Model file for the job. Use its own axes, mm. Face numbers are marked on the shaded views. A direction names the side the tool comes from. Round coordinates to 2 decimals unless told otherwise and drop trailing zeros. Write each loop counter-clockwise with the first axis right and the second up, starting at its lowest first coordinate (ties: lowest second). Pieces come first, ordered by that corner, then holes.
```python
from build123d import *

# Parameters (mm, degrees)
F0_W     = 50.8
F0_H     = 88.9
F1_DEPTH = 101.6
F2_W     = 50.8
F2_H     = 19.05
F3_DEPTH = 63.5
F4_W     = 50.8
F4_H     = 6.9018518552
F5_DEPTH = 50.8
F6_R     = 5.08


with BuildPart() as f1:
    # F0 (on Top) → F1 (new body)
    with BuildSketch(Plane.XY):
        Rectangle(F0_W, F0_H)
    extrude(amount=F1_DEPTH)

    # F2 (on face) → F3 (cut)
    with BuildSketch(Plane.XY.offset(101.6)):
        with Locations((0, -34.925)):
            Rectangle(F2_W, F2_H)
        with Locations((0, 34.925)):
            Rectangle(F2_W, F2_H)
    extrude(amount=-F3_DEPTH, mode=Mode.SUBTRACT)

    # F4 (on face) → F5 (cut)
    with BuildSketch(Plane.YZ.offset(25.4)):
        with Locations((0, 3.4509259276)):
            Rectangle(F4_W, F4_H)
    extrude(amount=-F5_DEPTH, mode=Mode.SUBTRACT)

    # F6
    f6_edges = [f1.edges().sort_by_distance(p)[0] for p in [
        (0, -25.4, 101.6),
        (-25.4, 0, 101.6),
        (0, 25.4, 101.6),
        (25.4, 0, 101.6),
        (25.4, -25.4, 69.85),
        (25.4, 25.4, 69.85),
        (-25.4, 25.4, 69.85),
        (-25.4, -25.4, 69.85),
        (0, -44.45, 38.1),
        (0, 44.45, 38.1),
    ]]
    fillet(f6_edges, radius=F6_R)


solid = f1.part
```
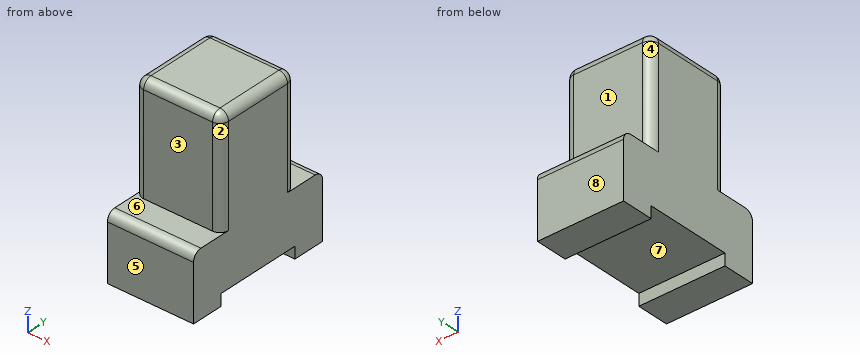
1) Wall check: probe 1 along Y at (x, z) = (-4, 4); probe 2 along Z at (x, y) = (-18, -6.5); probe 3 along Z at (x, y) = (15.5, 32.5). Give the ranges that are in metal, low to high.
2) Cut at C-C on y = -15. List the corners of the cut face in (x, z).
3) Flat gauge pins, fed straight in: pin 1 Ø4 at (x, y) = (-17.5, 25.5) entering from +Z; pin 2 Ø5 at (x, y) = (16, 31) entering from -Z; pin 3 Ø2 at (x, z) = (-1, 65.5) entering from -Y; pin 4 Ø3 at (x, z) = (-13.5, 83.5) entering from +Y. Where does each tip first touch, or does it go through?
4) Cut at B-B on z = 41.5. List the corners of the cut face in (x, y).
5) Which spindle directions (+Z, -Z, +X, -X, +Y, -Y) get a long thin tool onto all of the face, cutting with end or side? Do the marked faces 1, 2, 3 and 4. Say none if no direction does.
6) Pull direction Y, two halves, no side cores. Call the marked faces 5, 6, 7 and 8: released by +Y, released by -Y, zero draft, split by the parting line, or undercut.
7) Cut at A-A on x = -6.5. List the corners of the cut face in (y, z), and give its area (3 significant figures).
8) Cut at D-D on y = -24. List the corners of the cut face in (x, z).
Result sheet:
1. probe 1: y = -44.45 to -25.4, 25.4 to 44.45
1. probe 2: z = 6.9 to 101.6
1. probe 3: z = 0 to 38.1
2. outline: (-25.4, 6.9) - (25.4, 6.9) - (25.4, 96.52) arc R5.08 ccw to (20.32, 101.6) - (-20.32, 101.6) arc R5.08 ccw to (-25.4, 96.52) - close
3. pin 1: stops at z = 100.48
3. pin 2: stops at z = 0
3. pin 3: stops at y = -25.4
3. pin 4: stops at y = 25.4
4. outline: (-25.4, -20.32) arc R5.08 ccw to (-20.32, -25.4) - (20.32, -25.4) arc R5.08 ccw to (25.4, -20.32) - (25.4, 20.32) arc R5.08 ccw to (20.32, 25.4) - (-20.32, 25.4) arc R5.08 ccw to (-25.4, 20.32) - close
5. face 1: +Z, +X, -X, +Y
5. face 2: +Z, +X, -Y
5. face 3: +Z, +X, -X, -Y
5. face 4: +Z, -X, +Y
6. face 5: released by -Y
6. face 6: zero draft
6. face 7: undercut
6. face 8: released by +Y
7. outline: (-44.45, 0) - (-25.4, 0) - (-25.4, 6.9) - (25.4, 6.9) - (25.4, 0) - (44.45, 0) - (44.45, 33.02) arc R5.08 ccw to (39.37, 38.1) - (25.4, 38.1) - (25.4, 96.52) arc R5.08 ccw to (20.32, 101.6) - (-20.32, 101.6) arc R5.08 ccw to (-25.4, 96.52) - (-25.4, 38.1) - (-39.37, 38.1) arc R5.08 ccw to (-44.45, 33.02) - close
7. area: 6,240 mm2
8. outline: (-25.4, 6.9) - (25.4, 6.9) - (25.4, 38.1) - (23.82, 38.1) - (23.82, 96.52) arc R3.5 ccw to (20.32, 100.02) - (-20.32, 100.02) arc R3.5 ccw to (-23.82, 96.52) - (-23.82, 38.1) - (-25.4, 38.1) - close
